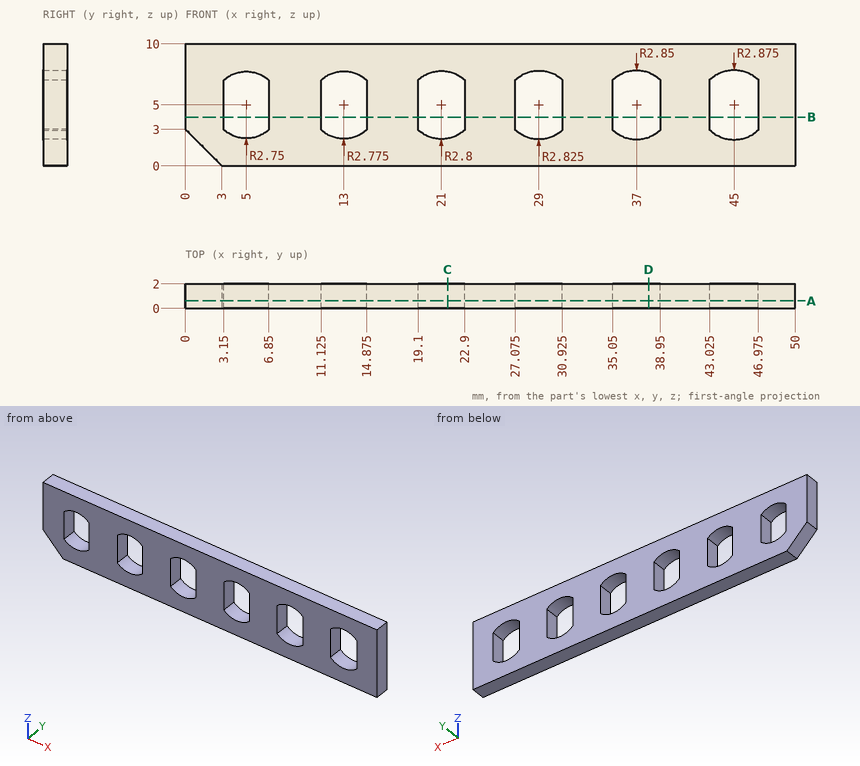
The drawing under review shows one solid part. Ordinate dimensions are in mm from its lowest x, y, z. Give positions to 0.01 mm unless a question says otherwise; leave off trailing zeros. Write each loop counter-clockwise with the first axis right and the second up, starting at its lowest first coordinate (ties: lowest second). Pieces come first, ordered by that corner, then holes. Notation, with made-up numbers: (-2, -7) -> (48, -7) arc R12 ccw to (48, 15) -> close; hole circle Ø9 at (-34, 37.5). An arc over 180 degrees is marked (long way). Put each result on its own line as item: value.
(1) We need section A-A, the plane y = 0.6. State how many separate pieces and enclosed holes the cut face has, and give its area (3 significant figures).
Results are:
separate pieces: 1
enclosed holes: 6
area: 377 mm²
(2) We need section D-D, the plane x = 38. Give the boundary of the cut face in (y, z).
Results are:
outline: (0, 0) -> (2, 0) -> (2, 2.33) -> (0, 2.33) -> close; (0, 7.67) -> (2, 7.67) -> (2, 10) -> (0, 10) -> close
(3) We need section C-C, the plane x = 21.5. Give the boundary of the cut face in (y, z) (3 decimals).
Results are:
outline: (0, 0) -> (2, 0) -> (2, 2.245) -> (0, 2.245) -> close; (0, 7.755) -> (2, 7.755) -> (2, 10) -> (0, 10) -> close
(4) To check wall thickness, follow probe 1 along Z at (x, y) = (44.5, 1.55); probe 2 along Z at (x, y) = (12, 0.75); probe 3 along X at (y, z) = (0.8, 2). State the ranges of each line that lie inside material, in increasing order. Write a range as from..to.
Results are:
probe 1: 0..2.17, 7.83..10
probe 2: 0..2.41, 7.59..10
probe 3: 1..50
(5) We need section B-B, the plane z = 4. Give the boundary of the cut face in (x, y) (3 decimals), and give its area (3 significant figures).
Results are:
outline: (0, 0) -> (3.15, 0) -> (3.15, 2) -> (0, 2) -> close; (6.85, 0) -> (11.125, 0) -> (11.125, 2) -> (6.85, 2) -> close; (14.875, 0) -> (19.1, 0) -> (19.1, 2) -> (14.875, 2) -> close; (22.9, 0) -> (27.075, 0) -> (27.075, 2) -> (22.9, 2) -> close; (30.925, 0) -> (35.05, 0) -> (35.05, 2) -> (30.925, 2) -> close; (38.95, 0) -> (43.025, 0) -> (43.025, 2) -> (38.95, 2) -> close; (46.975, 0) -> (50, 0) -> (50, 2) -> (46.975, 2) -> close
area: 54.1 mm²
